from build123d import *

# Parameters (mm, degrees)
SKETCH_1_R          = 16
SKETCH_1_R_2        = 7.75
SKETCH_1_R_3        = 1.7
EXTRUDE_1_DEPTH     = 4
SKETCH_2_R          = 7.75
EXTRUDE_2_DEPTH     = 7
CUT_EXTRUDE_START   = -11
SKETCH_3_W          = 1
SKETCH_3_H          = 8.04554885
SKETCH_3_H_2        = 6
CUT_EXTRUDE_1_DEPTH = 11
EXTRUDE_START       = -7
EXTRUDE_3_DEPTH     = 7
SKETCH_4_R          = 1.7
CUT_EXTRUDE_2_DEPTH = 8


with BuildPart() as part:
    # 草图1 → 凸台-拉伸1 (new body)
    with BuildSketch(Plane(origin=(0, 0, 0), x_dir=(1, 0, 0), z_dir=(0, 1, 0))):
        with Locations(Location((0, 0, 0), (0, 0, 270))):
            Circle(SKETCH_1_R)
        with Locations(Location((0, 0, 0), (0, 0, 270))):
            Circle(SKETCH_1_R_2, mode=Mode.SUBTRACT)
        with Locations(Location((0, 12.5, 0), (0, 0, 270))):
            Circle(SKETCH_1_R_3, mode=Mode.SUBTRACT)
        with Locations(Location((10.825317547, 6.25, 0), (0, 0, 270))):
            Circle(SKETCH_1_R_3, mode=Mode.SUBTRACT)
        with Locations(Location((10.825317547, -6.25, 0), (0, 0, 270))):
            Circle(SKETCH_1_R_3, mode=Mode.SUBTRACT)
        with Locations(Location((0, -12.5, 0), (0, 0, 270))):
            Circle(SKETCH_1_R_3, mode=Mode.SUBTRACT)
        with Locations(Location((-10.825317547, -6.25, 0), (0, 0, 270))):
            Circle(SKETCH_1_R_3, mode=Mode.SUBTRACT)
        with Locations(Location((-10.825317547, 6.25, 0), (0, 0, 270))):
            Circle(SKETCH_1_R_3, mode=Mode.SUBTRACT)
    extrude(amount=EXTRUDE_1_DEPTH)

    # 草图2 → 凸台-拉伸2 (add)
    with BuildSketch(Plane(origin=(0, 4, 0), x_dir=(1, 0, 0), z_dir=(0, 1, 0))):
        with BuildLine():
            ThreePointArc((-3.185514087, -11.05), (0, -9), (3.185514087, -11.05))
            ThreePointArc((3.185514087, -11.05), (6.555617772, -9.448485362), (9.23558726, -6.852293628))
            ThreePointArc((9.23558726, -6.852293628), (9.353074361, -5.4), (10.552053986, -4.572106372))
            ThreePointArc((10.552053986, -4.572106372), (11.260519989, -2.334671193), (11.5, 0))
            ThreePointArc((11.5, 0), (11.415272318, 1.393397971), (11.162337755, 2.766263876))
            ThreePointArc((11.162337755, 2.766263876), (7.794228634, 4.5), (7.976823668, 8.283736124))
            ThreePointArc((7.976823668, 8.283736124), (4.904819465, 10.401574209), (1.316466726, 11.4244))
            ThreePointArc((1.316466726, 11.4244), (0, 10.8), (-1.316466726, 11.4244))
            ThreePointArc((-1.316466726, 11.4244), (-4.904819465, 10.401574209), (-7.976823668, 8.283736124))
            ThreePointArc((-7.976823668, 8.283736124), (-7.492171243, 7.317771376), (-7.325317547, 6.25))
            ThreePointArc((-7.325317547, 6.25), (-8.472613861, 3.658709711), (-11.162337755, 2.766263876))
            ThreePointArc((-11.162337755, 2.766263876), (-11.460437236, -0.953088847), (-10.552053986, -4.572106372))
            ThreePointArc((-10.552053986, -4.572106372), (-9.530221401, -5.148761619), (-9.125317547, -6.25))
            ThreePointArc((-9.125317547, -6.25), (-9.153112194, -6.556152341), (-9.23558726, -6.852293628))
            ThreePointArc((-9.23558726, -6.852293628), (-6.555617772, -9.448485362), (-3.185514087, -11.05))
        make_face()
        with Locations(Location((0, 0, 0), (0, 0, 270))):
            Circle(SKETCH_2_R, mode=Mode.SUBTRACT)
    extrude(amount=EXTRUDE_2_DEPTH)

    # 草图3 → 切除-拉伸1 (cut)
    with BuildSketch(Plane(origin=(0, 11, 0), x_dir=(1, 0, 0), z_dir=(0, 1, 0)).offset(CUT_EXTRUDE_START)):
        with BuildLine():
            Line((0.5, -7.733854149), (0.5, 0))
            Line((0.5, 0), (-0.5, 0))
            Line((-0.5, 0), (-0.5, -7.733854149))
            ThreePointArc((-0.5, -7.733854149), (0, -7.75), (0.5, -7.733854149))
        make_face()
        with BuildLine():
            Line((-0.5, 0), (0.5, 0))
            Line((0.5, 0), (0.5, 7.733854149))
            ThreePointArc((0.5, 7.733854149), (0, 7.75), (-0.5, 7.733854149))
            Line((-0.5, 7.733854149), (-0.5, 0))
        make_face()
        with Locations((0, 20.977225575)):
            Rectangle(SKETCH_3_W, SKETCH_3_H)
        with Locations((0, 13.95445115)):
            Rectangle(SKETCH_3_W, SKETCH_3_H_2)
        with BuildLine():
            ThreePointArc((-0.5, 7.733854149), (0, 7.75), (0.5, 7.733854149))
            Line((0.5, 7.733854149), (0.5, 10.875192319))
            ThreePointArc((0.5, 10.875192319), (0, 10.8), (-0.5, 10.875192319))
            Line((-0.5, 10.875192319), (-0.5, 7.733854149))
        make_face()
    extrude(amount=CUT_EXTRUDE_1_DEPTH, mode=Mode.SUBTRACT)

    # 草图3<3> → 凸台-拉伸3 (add)
    with BuildSketch(Plane(origin=(0, 11, 0), x_dir=(1, 0, 0), z_dir=(0, 1, 0)).offset(EXTRUDE_START)):
        with BuildLine():
            Line((-0.708010418, 10.95445115), (-0.5, 10.95445115))
            Line((-0.5, 10.95445115), (-0.5, 16.95445115))
            Line((-0.5, 16.95445115), (-3.5, 16.95445115))
            Line((-3.5, 16.95445115), (-3.5, 10.95445115))
            ThreePointArc((-3.5, 10.95445115), (-2.419669587, 11.242561945), (-1.316466726, 11.4244))
            ThreePointArc((-1.316466726, 11.4244), (-1.039153457, 11.154578099), (-0.708010418, 10.95445115))
        make_face()
        with BuildLine():
            Line((0.5, 16.95445115), (0.5, 10.95445115))
            Line((0.5, 10.95445115), (0.708010418, 10.95445115))
            ThreePointArc((0.708010418, 10.95445115), (1.039153457, 11.154578099), (1.316466726, 11.4244))
            ThreePointArc((1.316466726, 11.4244), (2.419669587, 11.242561945), (3.5, 10.95445115))
            Line((3.5, 10.95445115), (3.5, 16.95445115))
            Line((3.5, 16.95445115), (0.5, 16.95445115))
        make_face()
        with BuildLine():
            ThreePointArc((-0.708010418, 10.95445115), (-0.605303877, 10.911413453), (-0.5, 10.875192319))
            Line((-0.5, 10.875192319), (-0.5, 10.95445115))
            Line((-0.5, 10.95445115), (-0.708010418, 10.95445115))
        make_face()
        with BuildLine():
            Line((0.5, 10.95445115), (0.5, 10.875192319))
            ThreePointArc((0.5, 10.875192319), (0.605303877, 10.911413453), (0.708010418, 10.95445115))
            Line((0.708010418, 10.95445115), (0.5, 10.95445115))
        make_face()
    extrude(amount=EXTRUDE_3_DEPTH)

    # 草图4 → 切除-拉伸2 (cut)
    with BuildSketch(Plane(origin=(3.5, 0, 0), x_dir=(0, 0, -1), z_dir=(1, 0, 0))):
        with Locations((13.95445115, 7)):
            Circle(SKETCH_4_R)
    extrude(amount=-CUT_EXTRUDE_2_DEPTH, mode=Mode.SUBTRACT)


solid = part.part
Work out the finished part from the listing and answer in its coordinate system (mm). A direction names the side the tool comes from. Give positions to 0.01 mm unless a question says otherwise; leave off trailing zeros. Order: outer loops, then holes, each group sorted by start corner. A loop starts at its lowest first (then second) coordinate and runs counter-clockwise, first axis right, second up. Notation, with made-up numbers: (-23, 86) - (27, 86) arc R18 cw to (27, 90) - close; hole circle Ø4 at (64.25, 76). An arc over 180 degrees is marked (long way). Answer as CSV lines item,"result". Start each with the question number.
Q1. The part is cut by section D-D (z = 12.5). Write down the section's boundary in (x, y).
Q2. Find the intervals of material crossed by L1, parallel to X at y = 2.2, z = 6.25; L2, parallel to X at y = 0.5, z = 5; L3, parallel to Z at x = -11.5, y = 3.75, in increasing order. Write a range as [from, to].
Q3. The mould has two halves that part along X. Classify faces 1 (the face through (1, 4, -13)), 2 (the face through (5.92, 7.45, -9.86)), 3 (the face through (-2, 4, -16.4)): +X half, -X half, draft (parallel to the pull), parting line (faces both ways), or undercut.
Q4. Given pin 1 Ø1.8 at (y, z) = (8, -15.5) entering from +X; pin 2 Ø1 at (x, z) = (-2.5, 11) entering from +Y; pin 3 Ø2 at (y, z) = (7, -13.95) entering from +X; pin 4 Ø5 at (y, z) = (7.5, -15) entering from -X, each flat-ended and moving along its own axis, determine where each tip first touches the part or whether it passes through.
Q5. The part is cut by section A-A (x = 0). Write down the section's boundary in (y, z).
Q6. For faces 4 (the face through (-11.465, 7.451, 0.901)), 5 (the face through (-1.7, 2, -12.5)), 6 (the face through (-0.5, 5, -12)), 7 (the face through (0, 7, 9)), 8 (the face through (3.5, 9, -14)), determine the directions among +Z, -Z, +X, -X, +Y, -Y from which every point of the face is accessible in a straight line to the end or side of a thin tool.
Q7. The part is cut by section B-B (z = 5.5). Write down the section's boundary in (x, y), then the cut area to 3 significant figures.
Q8. The part is cut by section C-C (y = 7). Write down the section's boundary in (x, z), then the cut area to 3 significant figures.
Check result:
1,outline,"(-9.99, 0) - (-1.7, 0) - (-1.7, 4) - (-9.99, 4) - close; (1.7, 0) - (9.99, 0) - (9.99, 4) - (1.7, 4) - close"
2,L1,"x = [-14.73, -12.53], [-9.13, -4.58], [4.58, 9.13], [12.53, 14.73]"
2,L2,"x = [-15.2, -11.98], [-9.67, -5.92], [5.92, 9.67], [11.98, 15.2]"
2,L3,"z = [-11.12, -7.81], [-4.69, 4.69], [7.81, 11.12]"
3,face 1,"undercut"
3,face 2,"+X half"
3,face 3,"draft"
4,pin 1,"stops at x = 3.5"
4,pin 2,"stops at y = 4"
4,pin 3,"passes through"
4,pin 4,"stops at x = -3.5"
5,outline,"(0, 7.75) - (11, 7.75) - (11, 9) - (4, 9) - (4, 10.8) - (0, 10.8) - close; (0, 14.2) - (4, 14.2) - (4, 16) - (0, 16) - close"
6,face 4,"-X, +Y"
6,face 5,"-Y"
6,face 6,"-Z, +Y, -Y"
6,face 7,"+Z, +Y"
6,face 8,"-Z, +X, +Y"
7,outline,"(-15.02, 0) - (-12.35, 0) - (-12.35, 4) - (-15.02, 4) - close; (-9.3, 0) - (-5.46, 0) - (-5.46, 11) - (-9.3, 11) - close; (5.46, 0) - (9.3, 0) - (9.3, 11) - (5.46, 11) - close; (12.35, 0) - (15.02, 0) - (15.02, 4) - (12.35, 4) - close"
7,area,"106 mm²"
8,outline,"(-11.16, -2.77) arc R3.5 cw to (-7.98, -8.28) arc R11.5 ccw to (-3.5, -10.95) - (-3.5, -12.25) - (-0.5, -12.25) - (-0.5, -7.73) arc R7.75 cw (long way) to (0.5, -7.73) - (0.5, -12.25) - (3.5, -12.25) - (3.5, -10.95) arc R11.5 ccw to (7.98, -8.28) arc R3.5 cw to (11.16, -2.77) arc R11.5 ccw to (10.55, 4.57) arc R1.7 cw to (9.24, 6.85) arc R11.5 ccw to (3.19, 11.05) arc R3.5 cw to (-3.19, 11.05) arc R11.5 ccw to (-9.24, 6.85) arc R1.7 cw to (-10.55, 4.57) arc R11.5 ccw to start; (-3.5, -16.95) - (-0.5, -16.95) - (-0.5, -15.65) - (-3.5, -15.65) - close; (0.5, -16.95) - (3.5, -16.95) - (3.5, -15.65) - (0.5, -15.65) - close"
8,area,"200 mm²"
